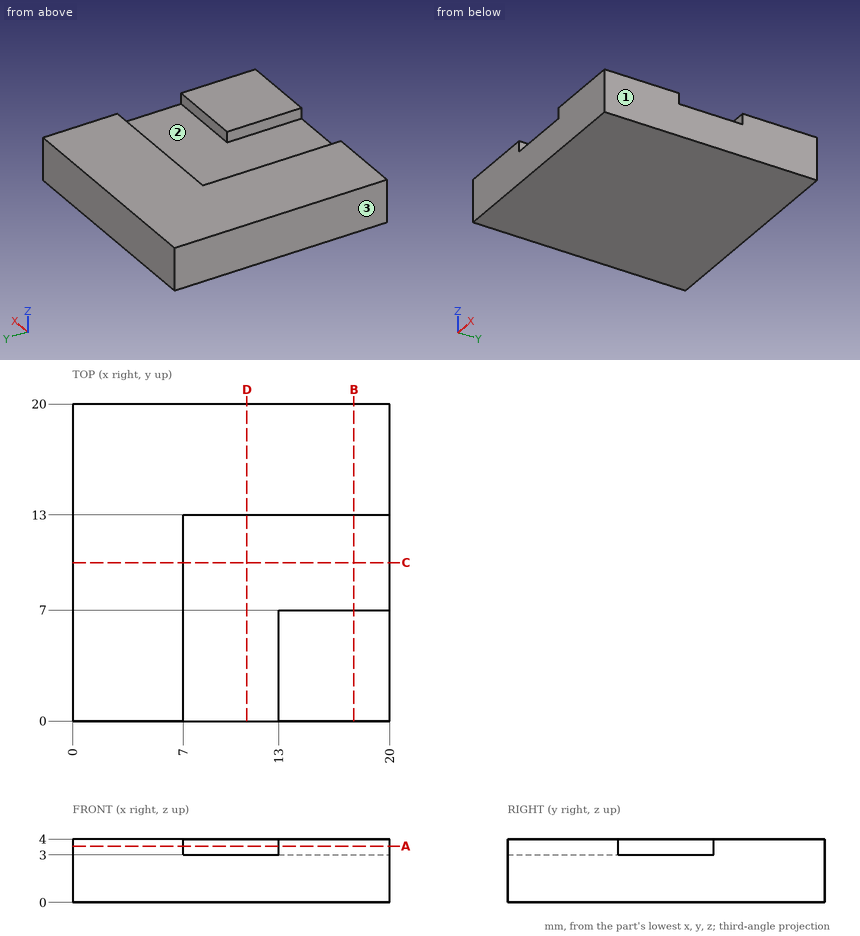
Check sheet for the drawn part. Datum: minimum x, y, z corner. Units: mm. Give positions to 0.01 mm unless a question says otherwise; leave off trailing zeros. Loops run counter-clockwise (first coordinate to the right, second up) from the corner with the lowest first, then second, coordinate; pieces in that order, holes last.
1) Sectioned sample at B-B, the plane x = 17.75. Enter the section's corners in (y, z).
2) Thickness scan on line 1 along X through (y, z) = (3, 3.55); line 2 along Z through (x, y) = (16.5, 8.25); line 3 along Y through (x, z) = (7.25, 3.55). Record the ranges inside material, lowest first.
3) Draft check along X on the marked faces 1, 2 and 3. Enter one of: pulls with the +X half, pulls with the -X half, needs draft (parallel to the pull), parting line crosses it, or undercut.
4) Sectioned sample at C-C, the plane y = 10. Enter the section's corners in (x, z).
5) Sectioned sample at A-A, the plane z = 3.55. Enter the section's corners in (x, y), then the cut area to 3 significant figures.
6) Sectioned sample at D-D, the plane x = 11. Enter the section's corners in (y, z), then the cut area to 3 significant figures.
Answers:
1. outline: (0, 0) - (20, 0) - (20, 4) - (13, 4) - (13, 3) - (7, 3) - (7, 4) - (0, 4) - close
2. line 1: x = 0 to 7, 13 to 20
2. line 2: z = 0 to 3
2. line 3: y = 13 to 20
3. face 1: pulls with the +X half
3. face 2: undercut
3. face 3: pulls with the -X half
4. outline: (0, 0) - (20, 0) - (20, 3) - (7, 3) - (7, 4) - (0, 4) - close
5. outline: (0, 0) - (7, 0) - (7, 13) - (20, 13) - (20, 20) - (0, 20) - close; (13, 0) - (20, 0) - (20, 7) - (13, 7) - close
5. area: 280 mm2
6. outline: (0, 0) - (20, 0) - (20, 4) - (13, 4) - (13, 3) - (0, 3) - close
6. area: 67.0 mm2
